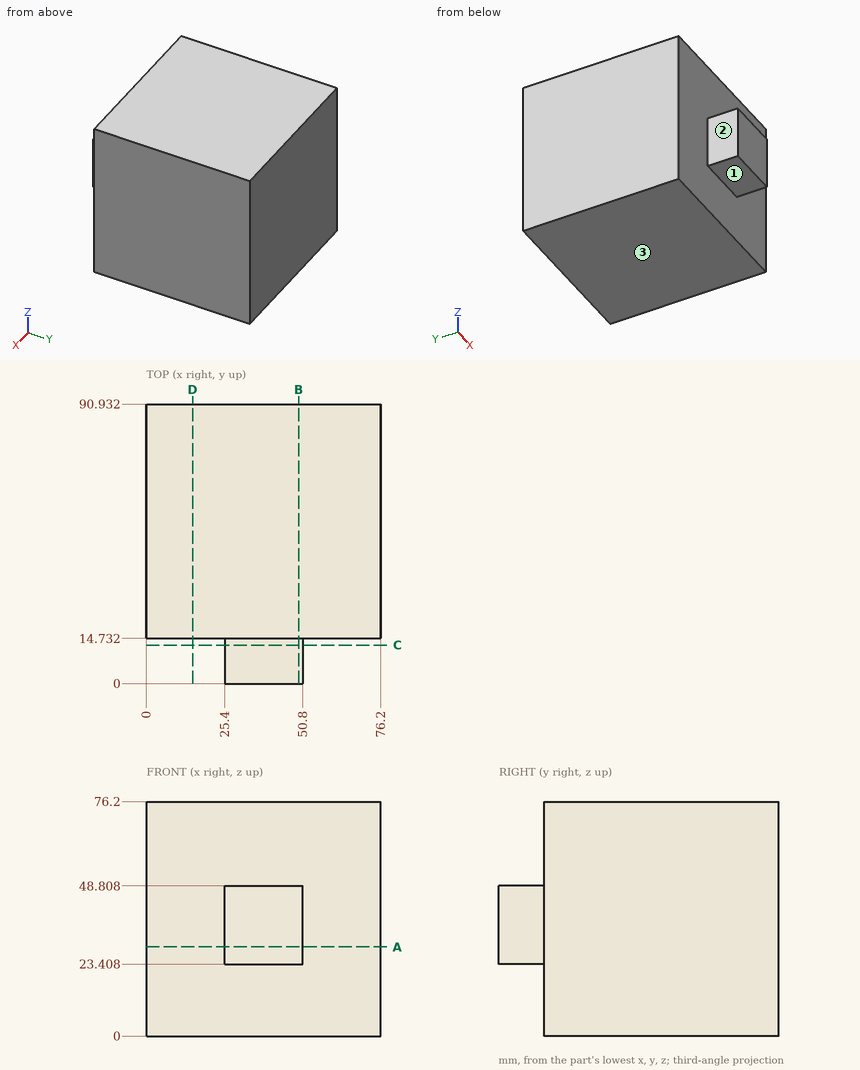
Here's the drawing with two shaded views (mm, measured from the low corner). I have some questions. A direction names the side the tool comes from. Give positions to 0.01 mm unless a question says otherwise; leave off trailing zeros. Order: outer loops, then holes, each group sorted by start corner. A loop starts at its lowest first (then second) coordinate and runs counter-clockwise, first axis right, second up. Notation, with made-up numbers: (-24.5, 36) - (2.5, 36) arc R22 cw to (2.5, 73) - close; hole circle Ø11 at (62.25, 76). An arc over 180 degrees is marked (long way). Use a Markdown table: item, result. Add a question column.
Q1. If we section it at D-D on x = 15: Write out the boundary of the cut face in (y, z).
Q2. If we section it at B-B on x = 49.5: Write out the boundary of the cut face in (y, z).
Q3. If we section it at A-A on z = 29: Write out the boundary of the cut face in (x, y).
Q4. Please list where these lines run through material, in increasing order: line 1 along Y through (x, z) = (27.5, 17.5); line 2 along X through (y, z) = (5, 27); line 3 along Z through (x, y) = (28, 14).
Q5. If we section it at C-C on y = 12.5: Write out the boundary of the cut face in (x, z).
Q6. On a 3-axis mill with a long thin cutter (end or side, diameter ignored), from which of +Z, -Z, +X, -X, +Y, -Y can I reach the whole of each face in a straight line? I mean the marked faces 1, 2 and 3. Say none if no direction works.
Q7. I'm going to push flat-ended pins straight in: pin 1 (4.5 mm diameter, centred on y = 9.5, z = 37, fed in from -X); pin 2 (4.5 mm diameter, centred on y = 6.5, z = 34.5, fed in from +X); pin 3 (4.5 mm diameter, centred on x = 41, y = 9.5, fed in from -Z); pin 4 (1.5 mm diameter, centred on x = 8, y = 72, fed in from -Z). Where does each tip first touch, or does it pass through?
Answers follow:
| question | item | result |
|---|---|---|
| 1 | outline | (14.73, 0) - (90.93, 0) - (90.93, 76.2) - (14.73, 76.2) - close |
| 2 | outline | (0, 23.41) - (14.73, 23.41) - (14.73, 0) - (90.93, 0) - (90.93, 76.2) - (14.73, 76.2) - (14.73, 48.81) - (0, 48.81) - close |
| 3 | outline | (0, 14.73) - (25.4, 14.73) - (25.4, 0) - (50.8, 0) - (50.8, 14.73) - (76.2, 14.73) - (76.2, 90.93) - (0, 90.93) - close |
| 4 | line 1 | y = 14.73 to 90.93 |
| 4 | line 2 | x = 25.4 to 50.8 |
| 4 | line 3 | z = 23.41 to 48.81 |
| 5 | outline | (25.4, 23.41) - (50.8, 23.41) - (50.8, 48.81) - (25.4, 48.81) - close |
| 6 | face 1 | -Z, +X, -X, -Y |
| 6 | face 2 | +Z, -Z, -X, -Y |
| 6 | face 3 | -Z, +X, -X, +Y, -Y |
| 7 | pin 1 | stops at x = 25.4 |
| 7 | pin 2 | stops at x = 50.8 |
| 7 | pin 3 | stops at z = 23.41 |
| 7 | pin 4 | stops at z = 0 |
